Source: three-view drawing plus pictorial views. Frame: mm from the lowest corner of the part. Give positions to 0.01 mm unless a question says otherwise; leave off trailing zeros. Loops run counter-clockwise (first coordinate to the right, second up) from the corner with the lowest first, then second, coordinate; pieces in that order, holes last.
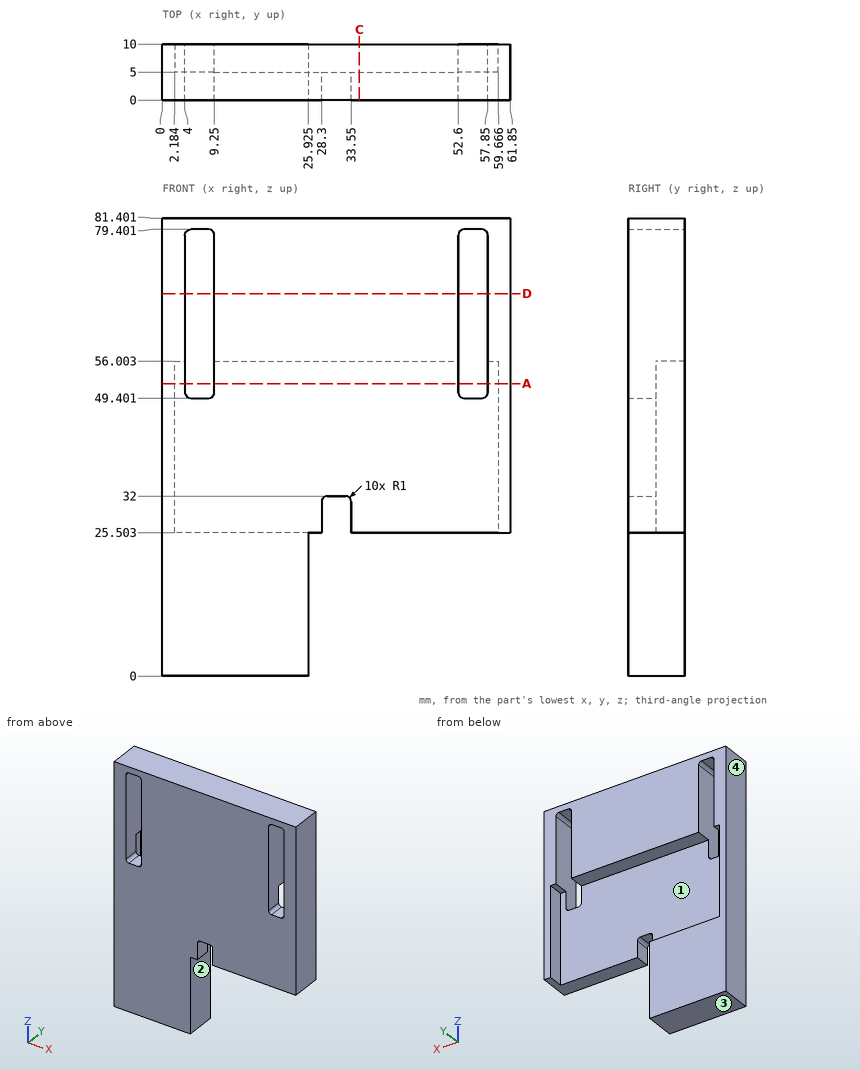
1) Ray query, probe 1 along X at (y, z) = (2.5, 56.5); probe 2 along Z at (x, y) = (57, 0.5); probe 3 along Z at (x, y) = (17, 5.25). Return the intervals inside material, ascending.
Checks:
probe 1: x = 0 to 4, 9.25 to 52.6, 57.85 to 61.85
probe 2: z = 25.5 to 49.41, 79.39 to 81.4
probe 3: z = 0 to 25.5, 56 to 81.4
2) Cut plane A-A (z = 52). State how many separate pieces and enclosed holes the cut face has.
Checks:
separate pieces: 3
enclosed holes: 0
3) Cut plane C-C (x = 35). Return loops of the section in (y, z).
Checks:
outline: (0, 25.5) - (5, 25.5) - (5, 56) - (10, 56) - (10, 81.4) - (0, 81.4) - close
4) Pull-direction query (X, two-part tool) for the marked faces 1, 2, 3 and 4; classes: released by +X, released by -X, zero draft, split by the parting line, or undercut.
Checks:
face 1: undercut
face 2: released by +X
face 3: zero draft
face 4: released by -X
5) Contact query for flat-ended pins moving along their axis: P1, Ø2, axis at x = 50, y = 5.5, coming from the -Z side; P2, Ø1, axis at x = 55.5, y = 7, coming from the -Z side; P3, Ø15.5, axis at x = 39, z = 37.5, coming from the +Y side. Output: stop coordinate, or through.
Checks:
P1: stops at z = 25.5
P2: stops at z = 79.4
P3: stops at y = 5
6) Cut plane D-D (z = 68). Return loops of the section in (x, y).
Checks:
outline: (0, 0) - (4, 0) - (4, 10) - (0, 10) - close; (9.25, 0) - (52.6, 0) - (52.6, 10) - (9.25, 10) - close; (57.85, 0) - (61.85, 0) - (61.85, 10) - (57.85, 10) - close
